Build history of the part. All positions in model axes, mm. Face numbers are marked on the shaded views. Round coordinates to 2 decimals unless told otherwise and drop trailing zeros. Write each loop counter-clockwise with the first axis right and the second up, starting at its lowest first coordinate (ties: lowest second). Pieces come first, ordered by that corner, then holes.
1) Saw through at B-B (z = 0). Write the cut outline in (x, y) (3 decimals).
2) Saw through at D-D (x = -15.5). Write the cut outline in (y, z).
3) Saw through at C-C (z = -19.5). Write the cut outline in (x, y), plus the area to 3 significant figures.
4) Saw through at A-A (x = 0). Write the cut outline in (y, z) (3 decimals).
5) Pull direction X, two halves, no side cores. Call the marked faces 1, 2, 3 and 4: +X half, -X half, draft (parallel to the pull), parting line (faces both ways), or undercut.
6) Wall check: probe 1 along Z at (x, y) = (0, -5.75) (3 decimals); probe 2 along Z at (x, y) = (-17, -16.5); probe 3 along Z at (x, y) = (-23.5, -10.5). Give the ranges that are in metal, low to high.
7) Flat gauge pins, fed straight in: pin 1 (2 mm diameter, centred on x = 11, y = -19.5, fed in from +Z); pin 2 (20 mm diameter, centred on x = 21.38, z = -11.96, fed in from -Y); pin 3 (4 mm diameter, centred on x = 31, y = -21, fed in from +Z); pin 4 (8 mm diameter, centred on x = 9, z = 32.5, fed in from +Y). Where does each tip first touch, or does it go through?
from build123d import *

# Parameters (mm, degrees)
F0_R     = 41.275
F0_R_2   = 10.9982
F1_DEPTH = 25.4


with BuildPart() as f1:
    # F0 (on Front) → F1 (new body)
    with BuildSketch(Plane.XZ):
        Circle(F0_R)
        with Locations((-20.721636, -11.962674)):
            Circle(F0_R_2, mode=Mode.SUBTRACT)
        with Locations((0, -27.447874)):
            Circle(F0_R_2, mode=Mode.SUBTRACT)
        with Locations((21.38141, -11.962674)):
            Circle(F0_R_2, mode=Mode.SUBTRACT)
        with Locations((-20.721636, 12.262576)):
            Circle(F0_R_2, mode=Mode.SUBTRACT)
        Circle(F0_R_2, mode=Mode.SUBTRACT)
        with Locations((20.518694, 12.77579)):
            Circle(F0_R_2, mode=Mode.SUBTRACT)
        with BuildLine():
            ThreePointArc((-2.430999, 34.840291), (0, 35.112324), (2.430999, 34.840291))
            ThreePointArc((2.430999, 34.840291), (8.593516, 30.977935), (10.9982, 24.114124))
            ThreePointArc((10.9982, 24.114124), (-6.86381, 15.520609), (-2.430999, 34.840291))
        make_face(mode=Mode.SUBTRACT)
    extrude(amount=F1_DEPTH)


solid = f1.part
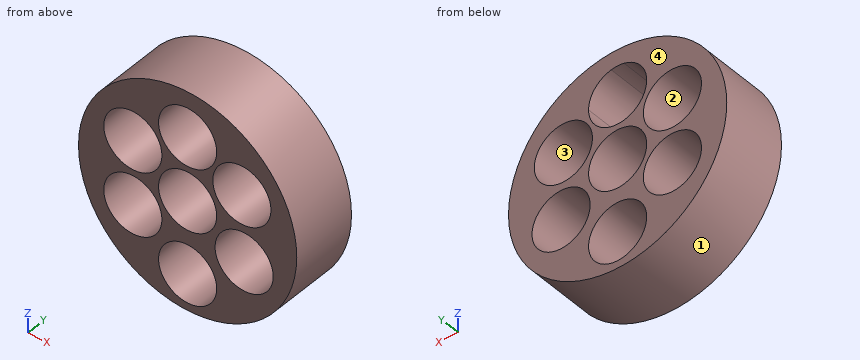
Evaluation:
1. outline: (-41.275, -25.4) - (-10.998, -25.4) - (-10.998, 0) - (-41.275, 0) - close; (10.998, -25.4) - (41.275, -25.4) - (41.275, 0) - (10.998, 0) - close
2. outline: (-25.4, -38.25) - (0, -38.25) - (0, -21.64) - (-25.4, -21.64) - close; (-25.4, -2.28) - (0, -2.28) - (0, 2.58) - (-25.4, 2.58) - close; (-25.4, 21.94) - (0, 21.94) - (0, 38.25) - (-25.4, 38.25) - close
3. outline: (-36.38, -25.4) - (-28.73, -25.4) - (-28.73, 0) - (-36.38, 0) - close; (-12.71, -25.4) - (-7.6, -25.4) - (-7.6, 0) - (-12.71, 0) - close; (7.6, -25.4) - (13.37, -25.4) - (13.37, 0) - (7.6, 0) - close; (29.39, -25.4) - (36.38, -25.4) - (36.38, 0) - (29.39, 0) - close
3. area: 648 mm2
4. outline: (-25.4, -41.275) - (0, -41.275) - (0, -38.446) - (-25.4, -38.446) - close; (-25.4, -16.45) - (0, -16.45) - (0, -10.998) - (-25.4, -10.998) - close; (-25.4, 10.998) - (0, 10.998) - (0, 13.116) - (-25.4, 13.116) - close; (-25.4, 35.112) - (0, 35.112) - (0, 41.275) - (-25.4, 41.275) - close
5. face 1: parting line
5. face 2: undercut
5. face 3: undercut
5. face 4: draft
6. probe 1: z = -41.275 to -38.446, -16.45 to -10.998, 10.998 to 13.116, 35.112 to 41.275
6. probe 2: z = -37.61 to -22.31, -1.61 to 1.91, 22.61 to 37.61
6. probe 3: z = -33.93 to -22.6, -1.32 to 1.62, 22.9 to 33.93
7. pin 1: stops at z = 40.05
7. pin 2: passes through
7. pin 3: stops at z = 29.37
7. pin 4: stops at y = 0
